Verification items for the finished model (mm, model axes). Coordinates: 2 decimals unless noted, no trailing zeros. Write each loop counter-clockwise with the first axis right and the second up, starting at its lowest first coordinate (ties: lowest second). Pieces come first, ordered by that corner, then holes. Notation, with made-up numbers: (41, 15.5) -> (48, 15.5) arc R11 ccw to (48, 36.5) -> close; hole circle Ø5 at (-32.5, 86). An arc over 180 degrees is marked (long way). Write item = value, one per line. Start each with the question number.
(1) Material ranges on probe 1 along X at (y, z) = (-1.15, 139.73) (3 decimals); probe 2 along X at (y, z) = (-1.75, 109) (3 decimals), recorded low to high. Write a range as [from, to].
(2) Section check A-A (z = 95.27). Record the cut outline in (x, y) (3 decimals), plus the area to 3 significant figures.
(3) Gauge pin test, flat end, axial feed: pin 1 Ø4.5 at (x, z) = (-7.874, 200.065) entering from +Y. Record the tip position at first contact, or that the pin passes through.
(4) Section check B-B (y = -2.7). State how many separate pieces and enclosed holes the cut face has, plus the area to 3 significant figures.
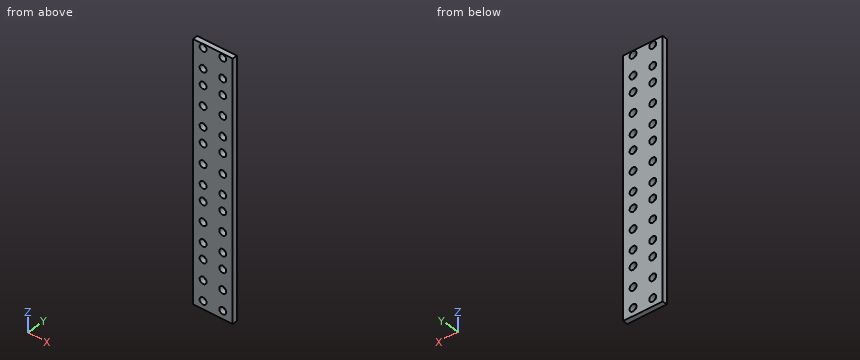
```python
from build123d import *

# Parameters (mm, degrees)
SKETCH_W         = 15.875
SKETCH_H         = 203.2
SKETCH_R         = 2.775
PAD_DEPTH        = 4
MIRROREDSKETCH_W = 15.875
MIRROREDSKETCH_H = 203.2
MIRROREDSKETCH_R = 2.775
PAD001_DEPTH     = 4


with BuildPart() as part:
    # Sketch → Pad (new body)
    with BuildSketch(Plane.XZ):
        with Locations((7.9375, 101.6)):
            Rectangle(SKETCH_W, SKETCH_H)
        with Locations((7.874, 6.35)):
            Circle(SKETCH_R, mode=Mode.SUBTRACT)
        with Locations((7.874, 22.23)):
            Circle(SKETCH_R, mode=Mode.SUBTRACT)
        with Locations((7.874, 38.11)):
            Circle(SKETCH_R, mode=Mode.SUBTRACT)
        with Locations((7.874, 50.81)):
            Circle(SKETCH_R, mode=Mode.SUBTRACT)
        with Locations((7.874, 66.69)):
            Circle(SKETCH_R, mode=Mode.SUBTRACT)
        with Locations((7.874, 82.57)):
            Circle(SKETCH_R, mode=Mode.SUBTRACT)
        with Locations((7.874, 95.27)):
            Circle(SKETCH_R, mode=Mode.SUBTRACT)
        with Locations((7.874, 111.15)):
            Circle(SKETCH_R, mode=Mode.SUBTRACT)
        with Locations((7.874, 127.03)):
            Circle(SKETCH_R, mode=Mode.SUBTRACT)
        with Locations((7.874, 139.73)):
            Circle(SKETCH_R, mode=Mode.SUBTRACT)
        with Locations((7.874, 155.61)):
            Circle(SKETCH_R, mode=Mode.SUBTRACT)
        with Locations((7.874, 171.49)):
            Circle(SKETCH_R, mode=Mode.SUBTRACT)
        with Locations((7.874, 184.19)):
            Circle(SKETCH_R, mode=Mode.SUBTRACT)
        with Locations((7.874, 200.065)):
            Circle(SKETCH_R, mode=Mode.SUBTRACT)
    extrude(amount=PAD_DEPTH)

    # MirroredSketch → Pad001 (join)
    with BuildSketch(Plane.XZ):
        with Locations((-7.9375, 101.6)):
            Rectangle(MIRROREDSKETCH_W, MIRROREDSKETCH_H)
        with Locations((-7.874, 6.35)):
            Circle(MIRROREDSKETCH_R, mode=Mode.SUBTRACT)
        with Locations((-7.874, 22.23)):
            Circle(MIRROREDSKETCH_R, mode=Mode.SUBTRACT)
        with Locations((-7.874, 38.11)):
            Circle(MIRROREDSKETCH_R, mode=Mode.SUBTRACT)
        with Locations((-7.874, 50.81)):
            Circle(MIRROREDSKETCH_R, mode=Mode.SUBTRACT)
        with Locations((-7.874, 66.69)):
            Circle(MIRROREDSKETCH_R, mode=Mode.SUBTRACT)
        with Locations((-7.874, 82.57)):
            Circle(MIRROREDSKETCH_R, mode=Mode.SUBTRACT)
        with Locations((-7.874, 95.27)):
            Circle(MIRROREDSKETCH_R, mode=Mode.SUBTRACT)
        with Locations((-7.874, 111.15)):
            Circle(MIRROREDSKETCH_R, mode=Mode.SUBTRACT)
        with Locations((-7.874, 127.03)):
            Circle(MIRROREDSKETCH_R, mode=Mode.SUBTRACT)
        with Locations((-7.874, 139.73)):
            Circle(MIRROREDSKETCH_R, mode=Mode.SUBTRACT)
        with Locations((-7.874, 155.61)):
            Circle(MIRROREDSKETCH_R, mode=Mode.SUBTRACT)
        with Locations((-7.874, 171.49)):
            Circle(MIRROREDSKETCH_R, mode=Mode.SUBTRACT)
        with Locations((-7.874, 184.19)):
            Circle(MIRROREDSKETCH_R, mode=Mode.SUBTRACT)
        with Locations((-7.874, 200.065)):
            Circle(MIRROREDSKETCH_R, mode=Mode.SUBTRACT)
    extrude(amount=PAD001_DEPTH)


solid = part.part
```
Response:
q1.probe_1 = [-15.875, -10.649], [-5.099, 5.099], [10.649, 15.875]
q1.probe_2 = [-15.875, -9.628], [-6.12, 6.12], [9.628, 15.875]
q2.outline = (-15.875, -4) -> (-10.649, -4) -> (-10.649, 0) -> (-15.875, 0) -> close; (-5.099, -4) -> (5.099, -4) -> (5.099, 0) -> (-5.099, 0) -> close; (10.649, -4) -> (15.875, -4) -> (15.875, 0) -> (10.649, 0) -> close
q2.area = 82.6 mm2
q3.pin_1 = through
q4.separate_pieces = 1
q4.enclosed_holes = 28
q4.area = 5,770 mm2
